Here's how the part is built. I have some questions about the finished solid (model axes, mm). A direction names the side the tool comes from. Give positions to 0.01 mm unless a question says otherwise; leave off trailing zeros. Loops run counter-clockwise (first coordinate to the right, second up) from the corner with the lowest first, then second, coordinate; pieces in that order, holes last. Notation, with made-up numbers: M 62.25,47 L 118.25,47 A19 ccw 118.25,84 Z; hole C -5.5,47 d10. An arc over 180 degrees is marked long. Answer as CSV lines item,"result". Start each with the question number.
Item 1: If I drill on line 1 along X through (y, z) = (1.5, -10); line 2 along Z through (x, y) = (-10.8, 1.15); line 3 along X through (y, z) = (15, -1.35), over which ranges is the centre line in solid material (lowest first)? Write a range as from..to.
Item 2: If we mould it in two halves opening along Y, with no side actions, what happens to faces 3 (the flat face through (0, 0, -10)), 4 (the cylindrical face through (-0.07, 16.5, -1.01)), 5 (the flat face through (0, 13, -2)), 6 (the flat face through (0, 30, -1))? For each: released by +Y, released by -Y, zero draft, split by the parting line, or undercut.
Item 3: I want a section at A-A on x = 0. List the corners of the cut face in (y, z) for me, plus the area to 3 significant figures.
Item 4: I want a section at B-B on z = -10. List the corners of the cut face in (x, y) for me, plus the area to 3 significant figures.
Item 5: Will these pins go through, and if not, where does the flat tip stop? P1, Ø4, axis at x = 0, y = 15, coming from the -Z side; P2, Ø8, axis at x = 12.5, z = -14.5, coming from the +Y side.
Item 6: I want a section at D-D on y = 22.75. List the corners of the cut face in (x, z) for me, plus the area to 3 significant figures.
Item 7: For faces 1 (the flat face through (0, 2, -11)), 2 (the cylindrical face through (11.7, 1, -8.8)), which set-ups out of +Z, -Z, +X, -X, +Y, -Y let a thin tool reach every point of the face, with its end or its side?
Item 8: I want a section at C-C on z = -6.25. List the corners of the cut face in (x, y) for me, plus the area to 3 significant figures.
Autodesk Inventor part; units mm, degrees
ref_plane "YZ Plane" through (0, 0, 0) normal (1, 0, 0) x (0, 1, 0)
ref_plane "XZ Plane" through (0, 0, 0) normal (0, 1, 0) x (-1, 0, 0)
ref_plane "XY Plane" through (0, 0, 0) normal (0, 0, 1) x (1, 0, 0)
sketch "Szkic1" plane through (0, 0, 0) normal (1, 0, 0) x (0, 1, 0)
  line L0 (2, 0) -> (30, 0)
  line L1 (30, 0) -> (30, -2)
  line L2 (30, -2) -> (2, -2)
  line L3 (2, 0) -> (0, 0)
  line L4 (0, 0) -> (0, -20)
  line L5 (0, -20) -> (2, -20)
  line L6 (2, -20) -> (2, -2)
  dimension "d2" = 2
  dimension "d7" = 30
  dimension "d8" = 20
  dimension "d9" = 2
extrude "Wyciągnięcie proste1" add sketch "Szkic1" along normal mid plane 37.6
sketch "Szkic2" plane through (-18.8, 0, 0) normal (0, 0, 1) x (1, 0, 0)
  line L0 (18.8, 0) -> (18.8, 15) construction
  dimension "d12" = 15
hole "Otwór1" at (0, 15, 0) direction (0, 0, -1) diameter 3 end through all
sketch "Szkic3" plane through (-18.8, 0, -20) normal (0, -1, 0) x (1, 0, 0)
  line L0 (0, 0) -> (0, 20)
  line L1 (37.6, 20) -> (37.6, 0)
  line L2 (0, 10) -> (8, 10) construction
  line L3 (37.6, 10) -> (29.6, 10) construction
  point P0 (18.8, 20)
  dimension "d20" = 8
  dimension "d21" = 8
hole "Otwór2" at (-10.8, 0, -10) at (10.8, 0, -10) direction (0, 1, 0) diameter 3 end through all
properties part number "bepf_podwozie_lacznik_glownego_wspornika" material "Aluminium 6061"
Result:
1,line 1,"-18.8..-12.3, -9.3..9.3, 12.3..18.8"
1,line 2,"-20..-11.5, -8.5..0"
1,line 3,"-18.8..-1.5, 1.5..18.8"
2,face 3,"released by -Y"
2,face 4,"undercut"
2,face 5,"zero draft"
2,face 6,"released by +Y"
3,outline,"M 0,-20 L 2,-20 L 2,-2 L 13.5,-2 L 13.5,0 L 0,0 Z; M 16.5,-2 L 30,-2 L 30,0 L 16.5,0 Z"
3,area,"90.0 mm^2"
4,outline,"M -18.8,0 L -12.3,0 L -12.3,2 L -18.8,2 Z; M -9.3,0 L 9.3,0 L 9.3,2 L -9.3,2 Z; M 12.3,0 L 18.8,0 L 18.8,2 L 12.3,2 Z"
4,area,"63.2 mm^2"
5,P1,"z = -2"
5,P2,"y = 2"
6,outline,"M -18.8,-2 L 18.8,-2 L 18.8,0 L -18.8,0 Z"
6,area,"75.2 mm^2"
7,face 1,"-Z, +X, -X, +Y"
7,face 2,"+Y, -Y"
8,outline,"M -18.8,0 L 18.8,0 L 18.8,2 L -18.8,2 Z"
8,area,"75.2 mm^2"
